Geometry: final body of the model. Coordinates: model frame, mm. A direction names the side the tool comes from. Round coordinates to 2 decimals unless told otherwise and drop trailing zeros. Write each loop counter-clockwise with the first axis right and the second up, starting at its lowest first coordinate (ties: lowest second). Pieces come first, ordered by that corner, then holes. Notation, with made-up numbers: (46.5, 64.5) - (86.5, 64.5) arc R18 ccw to (86.5, 74.5) - close; hole circle Ø7 at (14.25, -39.75). An arc over 180 degrees is marked (long way). Use a Markdown table: item, result. Add a question column.
Autodesk Inventor part; units mm, degrees
ref_plane "YZ Plane" through (0, 0, 0) normal (1, 0, 0) x (0, 1, 0)
ref_plane "XZ Plane" through (0, 0, 0) normal (0, 1, 0) x (-1, 0, 0)
ref_plane "XY Plane" through (0, 0, 0) normal (0, 0, 1) x (1, 0, 0)
sketch "Sketch1" plane through (0, 0, 0) normal (0, 0, 1) x (1, 0, 0)
  line L0 (7.88, 0) -> (2, 0)
  arc A0 (7.88, 0) -> (9.88, 2) centre (7.88, 2) ccw
  line L1 (9.88, 17.34) -> (9.88, 2)
  arc A1 (9.88, 17.34) -> (7.88, 19.34) centre (7.88, 17.34) ccw
  line L2 (2, 19.34) -> (7.88, 19.34)
  arc A2 (2, 19.34) -> (0, 17.34) centre (2, 17.34) ccw
  line L3 (0, 2) -> (0, 17.34)
  arc A3 (0, 2) -> (2, 0) centre (2, 2) ccw
  line L4 (0.47, 17.34) -> (0.47, 2)
  arc A4 (0.47, 2) -> (2, 0.47) centre (2, 2) ccw
  line L5 (2, 0.47) -> (7.88, 0.47)
  arc A5 (7.88, 0.47) -> (9.41, 2) centre (7.88, 2) ccw
  line L6 (9.41, 2) -> (9.41, 17.34)
  arc A6 (9.41, 17.34) -> (7.88, 18.87) centre (7.88, 17.34) ccw
  line L7 (7.88, 18.87) -> (2, 18.87)
  arc A7 (2, 18.87) -> (0.47, 17.34) centre (2, 17.34) ccw
  point P0 (0, 0)
  point P1 (0, 0)
  point P2 (0, 0)
  dimension "d0" = 0.47
extrude "Extrusion1" add sketch "Sketch1" along normal blind 13.5 contours A7 L7 A6 L6 A5 L5 A4 L4
sketch "Sketch2" plane through (0, 0, 0) normal (0, 0, -1) x (-1, 0, 0)
  arc A0 (-2, 0.47) -> (-0.47, 2) centre (-2, 2) ccw
  line L0 (-0.47, 17.34) -> (-0.47, 2)
  arc A1 (-0.47, 17.34) -> (-2, 18.87) centre (-2, 17.34) ccw
  line L1 (-7.88, 18.87) -> (-2, 18.87)
  arc A2 (-7.88, 18.87) -> (-9.41, 17.34) centre (-7.88, 17.34) ccw
  line L2 (-9.41, 2) -> (-9.41, 17.34)
  arc A3 (-9.41, 2) -> (-7.88, 0.47) centre (-7.88, 2) ccw
  line L3 (-2, 0.47) -> (-7.88, 0.47)
  arc A4 (-7.88, 20.37) -> (-10.91, 17.34) centre (-7.88, 17.34) ccw
  line L4 (-7.88, 20.37) -> (-2, 20.37)
  arc A5 (1.03, 17.34) -> (-2, 20.37) centre (-2, 17.34) ccw
  line L5 (1.03, 17.34) -> (1.03, 2)
  arc A6 (-2, -1.03) -> (1.03, 2) centre (-2, 2) ccw
  line L6 (-2, -1.03) -> (-7.88, -1.03)
  arc A7 (-10.91, 2) -> (-7.88, -1.03) centre (-7.88, 2) ccw
  line L7 (-10.91, 2) -> (-10.91, 17.34)
  point P0 (0, 0)
  dimension "d3" = 1.5
extrude "Extrusion2" add sketch "Sketch2" against normal blind 6
sketch "Sketch3" plane through (9.41, 2, 13.5) normal (1, 0, 0) x (0, 0, -1)
  line L0 (0, 0) -> (0, 15.34)
  line L1 (0, 7.67) -> (2, 7.67) construction
  line L2 (7.5, 16.87) -> (0, 16.87)
  line L3 (2, 7.67) -> (0, 16.87)
  line L4 (0, 0) -> (0, -1.53)
  line L5 (2, 7.67) -> (0, -1.53)
  line L6 (0, 16.87) -> (0, 15.34)
  line L7 (0, 16.87) -> (0, -1.53)
  point P0 (13.5, -2)
  dimension "d6" = 2
extrude "Extrusion3" cut sketch "Sketch3" against normal blind 9.175
sketch "Sketch4" plane through (0, 0, 6) normal (0, 0, 1) x (1, 0, 0)
  line L0 (9.41, 9.67) -> (0.47, 9.67)
  arc A0 (9.41, 17.34) -> (7.88, 18.87) centre (7.88, 17.34) ccw
  line L1 (7.88, 18.87) -> (2, 18.87)
  arc A1 (2, 18.87) -> (0.47, 17.34) centre (2, 17.34) ccw
  line L2 (0.47, 9.67) -> (0.47, 17.34)
  line L3 (9.41, 9.67) -> (0.47, 9.67)
  line L4 (9.41, 17.34) -> (9.41, 9.67)
  line L5 (13.6871, 9.67) -> (13.6871, 18.87)
  line L6 (4.94, 15.5745) -> (6.0697, 13.6177)
  line L7 (6.0697, 13.6177) -> (3.8103, 13.6177)
  line L8 (3.8103, 13.6177) -> (4.94, 15.5745)
  line L9 (-3.6206, 9.67) -> (18.3642, 9.67)
  line L10 (4.94, 3.7655) -> (6.0697, 5.7223)
  line L11 (6.0697, 5.7223) -> (3.8103, 5.7223)
  line L12 (3.8103, 5.7223) -> (4.94, 3.7655)
  point P0 (0, 0)
  point P1 (4.94, 9.67)
  point P2 (13.6871, 14.27)
  point P3 (4.94, 14.27)
  point P4 (4.94, 14.27)
  point P5 (4.94, 5.07)
  point P6 (4.94, 5.07)
extrude "Extrusion4" add sketch "Sketch4" along normal blind 10.7625 contours L6 L7 L8 | L12 L11 L10
sketch "Sketch5" plane through (9.41, 2, 6) normal (1, 0, 0) x (0, 0, -1)
  line L0 (-7.1674, 15.34) -> (-5.5, 7.67)
  line L1 (-5.5, 7.67) -> (-7.1674, 0)
  line L2 (-8.0469, 15.1488) -> (-6.421, 7.67)
  line L3 (-6.421, 7.67) -> (-8.0469, 0.1912)
  line L4 (-8.0469, 15.1488) -> (-12.9814, 15.34)
  line L5 (-12.9814, 15.34) -> (-12.7678, -1.5252)
  line L6 (-12.7678, -1.5252) -> (-8.0469, 0.1912)
  point P0 (6, -2)
  dimension "d11" = 0.9
extrude "Extrusion5" cut sketch "Sketch5" against normal blind 10.7625
sketch "Sketch6" plane through (0, 0, 0) normal (0, 0, -1) x (-1, 0, 0)
  line L0 (1.03, 17.34) -> (1.03, 2)
  line L1 (-2, -1.03) -> (-7.88, -1.03) construction
  line L2 (-9.41, 9.67) -> (-0.47, 9.67) construction
  line L3 (-9.88, 19.34) -> (0, 19.34) construction
  line L4 (0, 19.34) -> (0, 0) construction
  line L5 (0, 0) -> (-9.88, 0) construction
  line L6 (-9.88, 0) -> (-9.88, 19.34) construction
  line L7 (-9.88, 19.34) -> (0, 0) construction
  line L8 (0, 19.34) -> (-9.88, 0) construction
  line L9 (-0.47, 18.87) -> (-9.41, 18.87)
  line L10 (-9.41, 18.87) -> (-9.41, 0.47)
  line L11 (-9.41, 0.47) -> (-0.47, 0.47)
  line L12 (-0.47, 0.47) -> (-0.47, 18.87)
  point P0 (1.03, 9.67)
  point P1 (-4.94, -1.03)
  point P2 (-4.94, 9.67)
  dimension "d14" = 9.88
  dimension "d15" = 19.34
  dimension "d16" = 0.47
extrude "Extrusion6" add sketch "Sketch6" along normal blind 3
properties part number "IPC dumb rocker switch"
1) Section C-C, the plane y = 9. Return the cut outline in (x, z), then the cut area to 3 significant figures.
2) Set-up query: faces 1 (the flat face through (9.41, 10, 9)), 2 (the flat face through (4.367, 14.582, 13.022)), 3 (the flat face through (4.96, 4.98, 13.44)), 4 (the flat face through (0, 10, 6)), 5 (the flat face through (5, 0.47, 10)). Return all of +Z, -Z, +X, -X, +Y, -Y with unobstructed straight access to the full face (end or side cutting, diameter ignored); none if empty.
3) Section D-D, the plane y = 6. Return the cut outline in (x, z), then the cut area to 3 significant figures.
4) Material intervals for L1, parallel to Z at x = 0, y = 12.5; L2, parallel to Y at x = 3, z = -0.5; L3, parallel to Z at x = 6, y = 2, sorted ascending. Write a range as from..to.
5) Section A-A, the plane z = 4.25. Return the cut outline in (x, y).
6) Pin query (flat end, axial travel): P1, Ø3, axis at x = 6, z = 11, coming from the +Y side; P2, Ø0.9, axis at y = 8, z = -1, coming from the +X side; P3, Ø4.5, axis at x = 4.5, z = 9.5, coming from the -Y side. Return the tip coordinate at first contact, or that it passes through.
7) Draft query along Y for faces 6 (the flat face through (4.956, 14.392, 13.448)), 7 (the cylindrical face through (9.999, 19.506, 2.958)), 8 (the flat face through (10.91, 10, 3)), 9 (the flat face through (5.497, 4.73, 13.022)). Return one class per face: released by +Y, released by -Y, zero draft, split by the parting line, or undercut.
8) Section B-B, the plane x = 6.5. Return the cut outline in (y, z), then the cut area to 3 significant figures.
Output values:
| question | item | result |
|---|---|---|
| 1 | outline | (-1.03, 0) - (0.47, 0) - (0.47, -3) - (9.41, -3) - (9.41, 0) - (10.91, 0) - (10.91, 6) - (9.41, 6) - (9.41, 11.65) - (0.47, 11.65) - (0.47, 6) - (-1.03, 6) - close |
| 1 | area | 149 mm^2 |
| 2 | face 1 | +Z, +X, +Y, -Y |
| 2 | face 2 | +Z, -X |
| 2 | face 3 | +Z, +X, -X |
| 2 | face 4 | +Z |
| 2 | face 5 | +Z, +X, -X, -Y |
| 3 | outline | (-1.03, 0) - (0.47, 0) - (0.47, -3) - (9.41, -3) - (9.41, 0) - (10.91, 0) - (10.91, 6) - (9.41, 6) - (9.41, 12.3) - (0.47, 12.3) - (0.47, 6) - (-1.03, 6) - close |
| 3 | area | 155 mm^2 |
| 4 | L1 | z = 0..6 |
| 4 | L2 | y = 0.47..18.87 |
| 4 | L3 | z = -3..13.17 |
| 5 | outline | (-1.03, 2) arc R3.03 ccw to (2, -1.03) - (7.88, -1.03) arc R3.03 ccw to (10.91, 2) - (10.91, 17.34) arc R3.03 ccw to (7.88, 20.37) - (2, 20.37) arc R3.03 ccw to (-1.03, 17.34) - close |
| 6 | P1 | stops at y = 18.87 |
| 6 | P2 | stops at x = 9.41 |
| 6 | P3 | stops at y = 0.47 |
| 7 | face 6 | undercut |
| 7 | face 7 | released by +Y |
| 7 | face 8 | zero draft |
| 7 | face 9 | undercut |
| 8 | outline | (-1.03, 0) - (0.47, 0) - (0.47, -3) - (18.87, -3) - (18.87, 0) - (20.37, 0) - (20.37, 6) - (18.87, 6) - (18.87, 13.5) - (9.67, 11.5) - (0.47, 13.5) - (0.47, 6) - (-1.03, 6) - close |
| 8 | area | 303 mm^2 |
